from build123d import *

# Parameters (mm, degrees)
SKETCH1_W          = 122
SKETCH1_H          = 122
BASE_FLANGE1_DEPTH = 1.3
FILLET1_R          = 5
SKETCH3_R          = 2.5
CUT_EXTRUDE1_DEPTH = 10
SKETCH4_R          = 1.649999999
CUT_EXTRUDE2_DEPTH = 10


# Sheet-metal steps are written as plain solids
with BuildPart() as part:
    # Sketch1 → Base-Flange1 (new body)
    with BuildSketch(Plane(origin=(0, 0, 0), x_dir=(1, 0, 0), z_dir=(0, 1, 0))):
        Rectangle(SKETCH1_W, SKETCH1_H)
    extrude(amount=-BASE_FLANGE1_DEPTH)

    # Fillet1
    fillet1_edges = [part.edges().sort_by_distance(p)[0] for p in [
        (61, -0.65, 61),
        (-61, -0.65, 61),
        (-61, -0.65, -61),
        (61, -0.65, -61),
    ]]
    fillet(fillet1_edges, radius=FILLET1_R)

    # Sketch3 → Cut-Extrude1 (cut)
    with BuildSketch(Plane(origin=(0, 0, 0), x_dir=(1, 0, 0), z_dir=(0, 1, 0))):
        with Locations(Location((52.5, 52.5, 0), (0, 0, 270))):
            Circle(SKETCH3_R)
        with Locations(Location((-52.5, 52.5, 0), (0, 0, 270))):
            Circle(SKETCH3_R)
        with Locations(Location((-52.5, -52.5, 0), (0, 0, 270))):
            Circle(SKETCH3_R)
        with Locations(Location((52.5, -52.5, 0), (0, 0, 270))):
            Circle(SKETCH3_R)
    extrude(amount=-CUT_EXTRUDE1_DEPTH, mode=Mode.SUBTRACT)

    # Sketch4 → Cut-Extrude2 (cut)
    with BuildSketch(Plane(origin=(0, -1.3, 0), x_dir=(-1, 0, 0), z_dir=(0, -1, 0))):
        with Locations(Location((21.023848249, 36.422526924, 0), (0, 0, 90))):
            Circle(SKETCH4_R)
        with Locations(Location((21.023848249, 17.822526924, 0), (0, 0, 90))):
            Circle(SKETCH4_R)
        with Locations(Location((-16.576151751, 17.822526924, 0), (0, 0, 90))):
            Circle(SKETCH4_R)
        with Locations(Location((-16.576151751, 36.422526924, 0), (0, 0, 90))):
            Circle(SKETCH4_R)
    extrude(amount=-CUT_EXTRUDE2_DEPTH, mode=Mode.SUBTRACT)


solid = part.part
Read the model definition and answer for the solid it produces. Units are mm, in the model's axes. Give positions to 0.01 mm unless a question says otherwise; leave off trailing zeros. Loops run counter-clockwise (first coordinate to the right, second up) from the corner with the lowest first, then second, coordinate; pieces in that order, holes last. Notation, with made-up numbers: (54, 22) - (65, 22) arc R29 cw to (65, 49) - close; hole circle Ø4 at (40, -19). An arc over 180 degrees is marked (long way). Answer as CSV lines item,"result". Start each with the question number.
1) Straight lines are drawn through the part: L1, parallel to X at y = -0.5, z = -52.5; L2, parallel to X at y = -1, z = -18.5; L3, parallel to Z at x = 17.5, y = -0.2. For each, find the intervals that lie inside material, in ascending order. Write a range as from..to.
2) Find section A-A (x = -52.5). Write down the section's boundary in (y, z).
3) Each of these flat-tipped pins is pushed along its axis until it touches: pin 1 Ø4 at (x, z) = (52.5, -52.5) entering from +Y; pin 2 Ø2 at (x, z) = (-8, 40.5) entering from +Y. Where does it stop, or does it pass through?
4) Find section B-B (z = 52.5). Write down the section's boundary in (x, y).
5) Determine the mould class of faces 1 (the face through (51.54, -0.64, -50.19)), 2 (the face through (60, -1, -59)), 3 (the face through (-1, -1.3, -1)), 4 (the face through (-60, -1, -59)) for opening direction X: released by +X, released by -X, zero draft, split by the parting line, or undercut.
Findings below:
1,L1,"-61..-55, -50..50, 55..61"
1,L2,"-61..-22.53, -19.52..15.07, 18.08..61"
1,L3,"-61..-37.79, -35.06..-19.19, -16.46..61"
2,outline,"(-1.3, -61) - (0, -61) - (0, -55) - (-1.3, -55) - close; (-1.3, -50) - (0, -50) - (0, 50) - (-1.3, 50) - close; (-1.3, 55) - (0, 55) - (0, 61) - (-1.3, 61) - close"
3,pin 1,"through"
3,pin 2,"y = 0"
4,outline,"(-61, -1.3) - (-55, -1.3) - (-55, 0) - (-61, 0) - close; (-50, -1.3) - (50, -1.3) - (50, 0) - (-50, 0) - close; (55, -1.3) - (61, -1.3) - (61, 0) - (55, 0) - close"
5,face 1,"undercut"
5,face 2,"released by +X"
5,face 3,"zero draft"
5,face 4,"released by -X"
